Read the model definition and answer for the solid it produces. Units are mm, in the model's axes. A direction names the side the tool comes from. Give positions to 0.01 mm unless a question says otherwise; leave off trailing zeros. Loops run counter-clockwise (first coordinate to the right, second up) from the corner with the lowest first, then second, coordinate; pieces in that order, holes last. Notation, with made-up numbers: (63.5, -7.75) - (68.5, -7.75) arc R25 ccw to (68.5, 18.25) - close; hole circle Ø4 at (59.25, 37). An arc over 180 degrees is marked (long way). Use a Markdown table: item, result. Add a question column.
Item 1: A cutting plane is placed at A-A (y = 0). Determine the outline of the cut face in (x, z), plus the area to 3 significant figures.
Item 2: Consider probe 1 along Z at (x, y) = (-4.75, 0); probe 2 along Z at (x, y) = (5.25, 4.25); probe 3 along Y at (x, z) = (3.75, 0). Determine where each line is inside the solid, lowest interval first. Write a range as [from, to].
Item 3: Which of the six approach directions +Z, -Z, +X, -X, +Y, -Y give full straight-line access (tool end or side, diameter ignored) to faces 1 (the face through (-4.684, -8.563, -1.016)), 2 (the face through (-5, 7.8, 0)), 3 (the face through (-4.684, 5.162, -6.908)), 4 (the face through (-2.176, 3.356, -0.392)), 5 (the face through (-4.7, 3.4, 7.9))?
Item 4: A cutting plane is placed at D-D (z = 0). Give the number of separate pieces and of enclosed holes in the cut face, plus the area to 3 significant figures.
Item 5: For a pull along Z with two mould halves and no side action, classify faces 6 (the face through (-5, 0, -7.8)), 7 (the face through (4.503, 6.704, -3.194)), 8 (the face through (-4.684, 2.461, 9.124)), 9 (the face through (4.437, -9.915, 1.302)) as +Z half, -Z half, draft (parallel to the pull), parting line (faces both ways), or undercut.
Item 6: A cutting plane is placed at B-B (z = -5.5). Determine the outline of the cut face in (x, y).
Item 7: A cutting plane is placed at C-C (x = 7.5). Determine the outline of the cut face in (y, z).
Item 8: Each of these flat-tipped pins is pushed along its axis until it touches: P1, Ø5, axis at x = 2, z = 7.5, coming from the +Y side; P2, Ø1.5, axis at x = -3, y = 0.5, coming from the +Z side; P3, Ø1.1, axis at x = -6.5, z = 0, coming from the -Y side; P4, Ø4, axis at y = 6.5, z = 8, coming from the +X side. Where does it stop, or does it pass through?
Solid Edge part; units mm, degrees
sketch "Sketch1" plane through (0, 0, 0) normal (1, 0, 0) x (0, 1, 0)
  circle A0 centre (0, 0) radius 9.45
extrude "Protrusion1" add sketch "Sketch1" against normal blind 9.5
sketch "Sketch2" plane through (0, 0, 0) normal (1, 0, 0) x (0, 1, 0)
  circle A0 centre (0, 0) radius 4
extrude "Cutout1" cut sketch "Sketch2" against normal up to next
sketch "Sketch3" plane through (0, 0, 0) normal (1, 0, 0) x (0, 1, 0)
  line L0 (1.382, 9.3484) -> (0.66, 7.8)
  line L1 (0.66, 7.8) -> (-0.66, 7.8)
  line L2 (-0.66, 7.8) -> (-1.382, 9.3484)
  arc A0 (1.382, 9.3484) -> (-1.382, 9.3484) centre (0, 0) ccw
extrude "Cutout2" cut sketch "Sketch3" against normal blind 14000
pattern_circular "Pattern1" count 12 over 360 about axis through (0, 0, 0) along (1, 0, 0) of "Cutout2"
sketch "Sketch4" plane through (0, 0, 0) normal (1, 0, 0) x (0, -0.866, 0.5)
  line L0 (-3.9559, 0.5921) -> (-2.2252, -3.324)
  arc A0 (-2.2252, -3.3239) -> (-3.9559, 0.5921) centre (0, 0) cw
extrude "Protrusion2" add sketch "Sketch4" against normal up to vertex (9.5 mm away)
sketch "Sketch5" plane through (0, 0, 0) normal (1, 0, 0) x (0, -0.866, 0.5)
  line L0 (-3.9559, 0.5921) -> (-2.2252, -3.324)
  arc A0 (-2.2252, -3.3239) -> (-3.9559, 0.5921) centre (0, 0) cw
  circle A1 centre (0, 0) radius 10
  circle A2 centre (0, 0) radius 4
extrude "ExtrudedProtrusion_4" add sketch "Sketch5" along normal blind 9
sketch "Sketch6" plane through (0, 0, 0) normal (1, 0, 0) x (0, -0.866, 0.5)
  line L0 (-3.9559, 0.5921) -> (-2.2252, -3.324)
  arc A0 (-2.2252, -3.3239) -> (-3.9559, 0.5921) centre (0, 0) cw
extrude "Protrusion3" add sketch "Sketch6" along normal up to vertex (9 mm away)
hole "Hole_2" at (4.5559, 9.9488, -1.0824) direction (0, -0.9942, 0.1072) diameter 4.3 end up to next counterbore diameter 7.5 counterbore depth 3
properties material "Steel"
Geometry says:
| question | item | result |
|---|---|---|
| 1 | outline | (-9.5, -7.8) - (0, -7.8) - (0, -10) - (9, -10) - (9, -4) - (-9.5, -4) - close; (-9.5, 4) - (9, 4) - (9, 10) - (0, 10) - (0, 7.8) - (-9.5, 7.8) - close |
| 1 | area | 180 mm² |
| 2 | probe 1 | [-7.8, -4], [4, 7.8] |
| 2 | probe 2 | [-9.05, -2.51], [1.58, 9.05] |
| 2 | probe 3 | [-10, -4] |
| 3 | face 1 | -X, -Y |
| 3 | face 2 | -X, +Y |
| 3 | face 3 | -Z, -X |
| 3 | face 4 | +X, -X |
| 3 | face 5 | -X |
| 4 | separate pieces | 3 |
| 4 | enclosed holes | 0 |
| 4 | area | 155 mm² |
| 5 | face 6 | -Z half |
| 5 | face 7 | undercut |
| 5 | face 8 | +Z half |
| 5 | face 9 | parting line |
| 6 | outline | (-9.5, -7.15) - (0, -7.15) - (0, -8.35) - (9, -8.35) - (9, 8.35) - (0, 8.35) - (0, 7.15) - (-9.5, 7.15) - close |
| 7 | outline | (6.72, -3.07) - (7.22, 1.55) - (9.92, 1.26) arc R10 ccw (long way) to (9.42, -3.36) - close; hole (3.13, -2.49) - (3.59, 1.77) arc R4 ccw (long way) to start |
| 8 | P1 | y = 8.66 |
| 8 | P2 | z = 9.07 |
| 8 | P3 | y = -7.8 |
| 8 | P4 | x = 9 |
